Model file for the job. Use its own axes, mm. A direction names the side the tool comes from. Round coordinates to 2 decimals unless told otherwise and drop trailing zeros. Order: outer loops, then holes, each group sorted by start corner. A loop starts at its lowest first (then second) coordinate and runs counter-clockwise, first axis right, second up. Notation, with made-up numbers: (5.5, 67) -> (20.5, 67) arc R18 ccw to (20.5, 94) -> close; hole circle Ø11 at (-26, 38). An arc over 180 degrees is marked (long way). Put each result on its own line as item: value. Start each with the question number.
Q1. Cut at D-D, the plane z = -3.75. List the corners of the cut face in (x, y), and give its area (3 significant figures).
Q2. Probe L1, parallel to Y at x = -2.25, z = 0; L2, parallel to Y at x = -8.25, z = -0.25; L3, parallel to X at y = 9.25, z = -1. List the from-to ranges inside material, lowest first.
Q3. Cut at B-B, the plane z = 0. List the corners of the cut face in (x, y), and give its area (3 significant figures).
Q4. Flat gauge pins, fed straight in: P1, Ø5, axis at y = 4, z = 0, coming from the -X side; P2, Ø3, axis at x = -10.5, z = -0.5, coming from the -Y side; P3, Ø3, axis at y = 10, z = -2, coming from the +X side. Where does each tip first touch, or does it go through?
Q5. Pull direction Y, two halves, no side cores. Call faces 3 (the face through (-2, 22.5, 0)), 4 (the face through (-3.944, 9.536, 0.325)), 5 (the face through (-8, 7, 0)), 6 (the face through (-10, 15, 0)): released by +Y, released by -Y, zero draft, split by the parting line, or undercut.
Q6. Cut at A-A, the plane y = 4. List the corners of the cut face in (x, z).
Q7. Cut at C-C, the plane y = 11.75. List the corners of the cut face in (x, z).
Q8. 3-axis set-ups, long thin cutter, end or side, ignore diameter. For faces 1 (the face through (-11.5, 19, 0)), 2 (the face through (0, 8, 0)): which of +Z, -Z, +X, -X, +Y, -Y reach the whole face in a straight line?
Autodesk Inventor part; units mm, degrees
ref_plane "YZ Plane" through (0, 0, 0) normal (1, 0, 0) x (0, 1, 0)
ref_plane "XZ Plane" through (0, 0, 0) normal (0, 1, 0) x (-1, 0, 0)
ref_plane "XY Plane" through (0, 0, 0) normal (0, 0, 1) x (1, 0, 0)
sketch "Sketch1" plane through (0, 0, 0) normal (0, 0, 1) x (1, 0, 0)
  line L0 (0, 0) -> (-8, 0)
  line L1 (-8, 0) -> (-8, 15)
  line L2 (-8, 15) -> (0, 15)
  line L3 (0, 15) -> (0, 0)
  line L4 (8, 22.5) -> (-11.5, 22.5)
  line L5 (-11.5, 22.5) -> (-11.5, 15)
  line L6 (-11.5, 15) -> (8, 15)
  line L7 (8, 15) -> (8, 22.5)
  line L8 (0, 15) -> (1, 15)
  line L9 (0, 14) -> (0, 15)
  point P0 (0.5, 15)
  point P1 (0.5, 14)
  dimension "d0" = 15
  dimension "d1" = 1
  dimension "d3" = 19.5
  dimension "d4" = 3.5
  dimension "d5" = 8
  dimension "d6" = 7.5
extrude "Extrusion1" add sketch "Sketch1" along normal mid plane 10
sketch "Sketch2" plane through (0, 0, 5) normal (1, 0, 0) x (0, 0, -1)
  circle A0 centre (5, 4) radius 1.5
  circle A1 centre (5, 11) radius 1.5
  line L0 (10, 14) -> (0, 14)
  line L1 (10, 0) -> (0, 0)
  line L2 (10, 15) -> (0, 15)
  point P0 (5, 0)
  point P1 (5, 0)
  point P2 (5, 0)
  dimension "d9" = 3
  dimension "d10" = 3
  dimension "d12" = 7
  dimension "d19" = 4
extrude "Extrusion2" cut sketch "Sketch2" against normal through all
thread "Thread1"
thread "Thread2"
properties part number "Connector2"
Ans:
1. outline: (-11.5, 15) -> (-8, 15) -> (-8, 0) -> (0, 0) -> (0, 15) -> (8, 15) -> (8, 22.5) -> (-11.5, 22.5) -> close
1. area: 266 mm^2
2. L1: y = 0 to 2.5, 5.5 to 9.5, 12.5 to 22.5
2. L2: y = 15 to 22.5
2. L3: x = -8 to 0
3. outline: (-11.5, 15) -> (-8, 15) -> (-8, 12.5) -> (0, 12.5) -> (0, 15) -> (8, 15) -> (8, 22.5) -> (-11.5, 22.5) -> close; (-8, 0) -> (0, 0) -> (0, 2.5) -> (-8, 2.5) -> close; (-8, 5.5) -> (0, 5.5) -> (0, 9.5) -> (-8, 9.5) -> close
3. area: 218 mm^2
4. P1: stops at x = -8
4. P2: stops at y = 15
4. P3: stops at x = 0
5. face 3: released by +Y
5. face 4: undercut
5. face 5: zero draft
5. face 6: released by -Y
6. outline: (-8, -5) -> (0, -5) -> (0, -1.5) -> (-8, -1.5) -> close; (-8, 1.5) -> (0, 1.5) -> (0, 5) -> (-8, 5) -> close
7. outline: (-8, -5) -> (0, -5) -> (0, -1.3) -> (-8, -1.3) -> close; (-8, 1.3) -> (0, 1.3) -> (0, 5) -> (-8, 5) -> close
8. face 1: +Z, -Z, -X, +Y, -Y
8. face 2: +Z, -Z, +X, -Y
